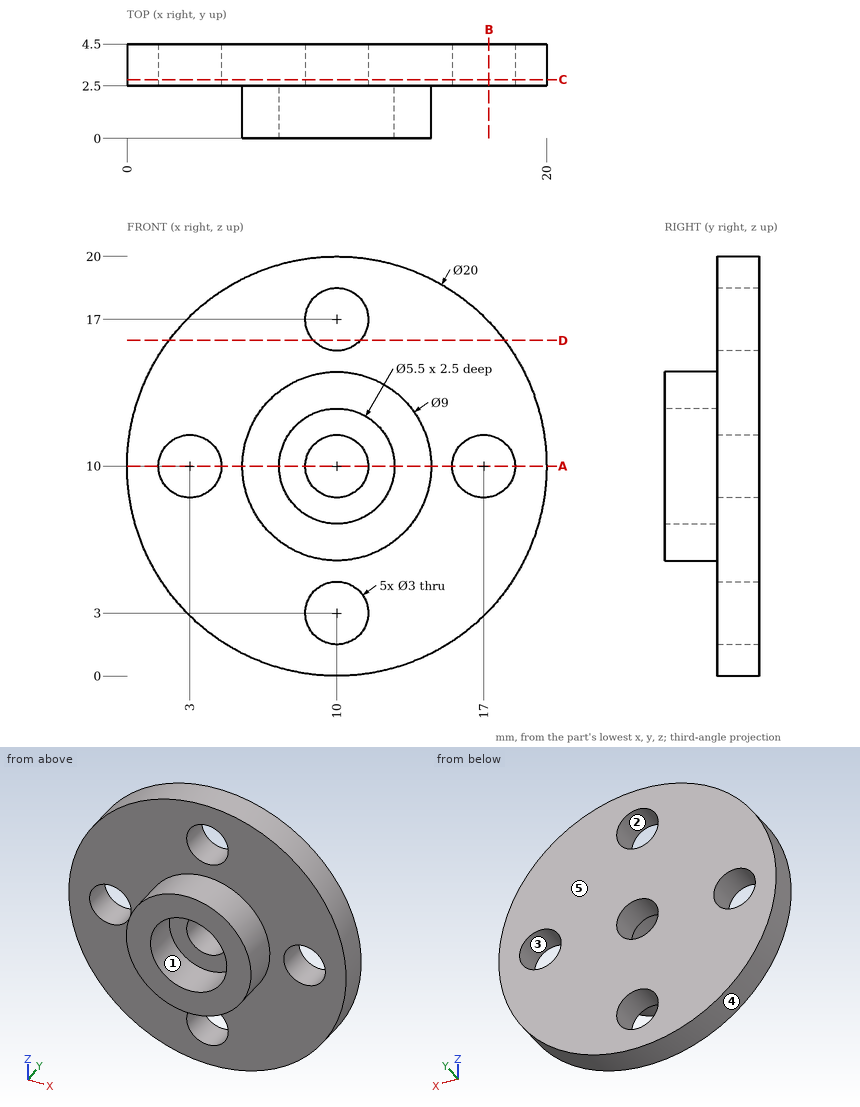
The figure shows three views and two pictorial views of one solid part (mm, origin at its lowest corner). Answer the questions. A direction names the side the tool comes from. Give positions to 0.01 mm unless a question says otherwise; leave off trailing zeros. Loops run counter-clockwise (first coordinate to the right, second up) from the corner with the lowest first, then second, coordinate; pieces in that order, holes last. Notation, with made-up numbers: (73, -39.75) - (104, -39.75) arc R26 cw to (104, -0.75) - close; hole circle Ø8 at (20.25, 62). An arc over 180 degrees is marked (long way). Use one line per item in the form item = value.
1. Which of the six approach directions +Z, -Z, +X, -X, +Y, -Y give full straight-line access (tool end or side, diameter ignored) to the marked faces 1 and 2?
Calculated:
face_1 = -Y
face_2 = +Y, -Y
2. Find the intervals of material crossed by line 1 along X through (y, z) = (3.75, 10); line 2 along Y through (x, z) = (18.75, 12.25); line 3 along Z through (x, y) = (15.75, 3.3), in increasing order. Write a range as [from, to].
Calculated:
line_1 = [0, 1.5], [4.5, 8.5], [11.5, 15.5], [18.5, 20]
line_2 = [2.5, 4.5]
line_3 = [1.82, 9.17], [10.83, 18.18]
3. Section A-A on z = 10 is taken. Give the vertices of the cut face in (x, y).
Calculated:
outline = (0, 2.5) - (1.5, 2.5) - (1.5, 4.5) - (0, 4.5) - close; (4.5, 2.5) - (5.5, 2.5) - (5.5, 0) - (7.25, 0) - (7.25, 2.5) - (8.5, 2.5) - (8.5, 4.5) - (4.5, 4.5) - close; (11.5, 2.5) - (12.75, 2.5) - (12.75, 0) - (14.5, 0) - (14.5, 2.5) - (15.5, 2.5) - (15.5, 4.5) - (11.5, 4.5) - close; (18.5, 2.5) - (20, 2.5) - (20, 4.5) - (18.5, 4.5) - close
4. Section D-D on z = 16 is taken. Give the vertices of the cut face in (x, y).
Calculated:
outline = (2, 2.5) - (8.88, 2.5) - (8.88, 4.5) - (2, 4.5) - close; (11.12, 2.5) - (18, 2.5) - (18, 4.5) - (11.12, 4.5) - close
5. Section C-C on y = 2.8 is taken. Give the vertices of the cut face in (x, z).
Calculated:
outline = circle Ø20 at (10, 10); hole circle Ø3 at (3, 10); hole circle Ø3 at (10, 3); hole circle Ø3 at (10, 10); hole circle Ø3 at (10, 17); hole circle Ø3 at (17, 10)
6. Given pin 1 Ø5 at (x, z) = (10, 10) entering from -Y; pin 2 Ø1.5 at (x, y) = (15, 2) entering from -Z; pin 3 Ø1 at (y, z) = (1.5, 9.5) entering from +X, each flat-ended and moving along its own axis, determine where each tip first touches the part or whether it passes through.
Calculated:
pin_1 = 2.5
pin_2 = 1.04
pin_3 = 14.5
7. The mould has two halves that part along Z. Classify the marked faces 3, 4 and 5: pulls with the +Z half, pulls with the -Z half, needs draft (parallel to the pull), parting line crosses it, or undercut.
Calculated:
face_3 = undercut
face_4 = parting line crosses it
face_5 = needs draft
8. Section B-B on x = 17.25 is taken. Give the vertices of the cut face in (y, z).
Calculated:
outline = (2.5, 3.11) - (4.5, 3.11) - (4.5, 8.52) - (2.5, 8.52) - close; (2.5, 11.48) - (4.5, 11.48) - (4.5, 16.89) - (2.5, 16.89) - close
